CAD build for the part. Positions are in the model's coordinates, mm. Face numbers are marked on the shaded views. A direction names the side the tool comes from. Round coordinates to 2 decimals unless told otherwise and drop trailing zeros. Loops run counter-clockwise (first coordinate to the right, second up) from the corner with the lowest first, then second, coordinate; pieces in that order, holes last. Notation, with made-up numbers: M 76.5,-1.75 L 107.5,-1.75 A7 ccw 107.5,6.25 Z; hole C -27,32 d8. An arc over 180 degrees is marked long. Use a Markdown table: item, result. Add a question column.
(1) Wall check: L1, parallel to Y at x = -15.25, z = 1.2; L2, parallel to Y at x = 5.5, z = 7.75; L3, parallel to Z at x = 8, y = 13. Give the ranges that are in metal, low to high.
(2) Band-saw the part on D-D, the plane y = -9.5. Write the cut outline in (x, z), and give its area (3 significant figures).
(3) Which spindle directions (+Z, -Z, +X, -X, +Y, -Y) get a long thin tool onto all of the face, cutting with end or side? Do the marked faces 1, 2 and 3. Say none if no direction does.
(4) Band-saw the part on A-A, the plane x = 6.5. Give the number of separate pieces and of enclosed holes in the cut face, and give its area (3 significant figures).
(5) Flat gauge pins, fed straight in: P1, Ø1.5, axis at x = 8, z = 3.5, coming from the -Y side; P2, Ø1.6, axis at x = 15, z = 7.5, coming from the +Y side; P3, Ø2.5, axis at x = 15.25, y = -15.25, coming from the +Z side; P4, Ø3, axis at y = 10, z = 7.5, coming from the +X side. Where does each tip first touch, or does it go through?
(6) Band-saw the part on C-C, the plane y = -15.25. Write the cut outline in (x, z), and give its area (3 significant figures).
(7) Band-saw the part on B-B, the plane x = -15.25. Write the cut outline in (y, z), and give its area (3 significant figures).
(8) Two-plate mould, pull along Y, no slides. Class the marked faces 4, 5 and 6: released by +Y, released by -Y, zero draft, split by the parting line, or undercut.
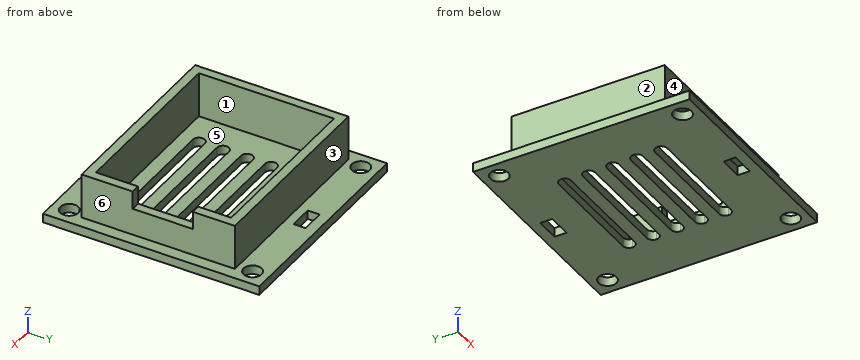
from build123d import *

# Parameters (mm, degrees)
F0_W      = 36
F0_H      = 36
F0_R      = 1.5
F3_DEPTH  = 1.5
F1_W      = 32
F1_H      = 25.5
F4_DEPTH  = 9
F5_T      = -1.5
F6_DEPTH  = 25
F7_W      = 1.5
F7_H      = 10
F8_DEPTH  = 3
F9_W      = 4
F9_H      = 2
F10_DEPTH = 25


with BuildPart() as f3:
    # F0 (on Top) → F3 (new body)
    with BuildSketch(Plane.XY):
        Rectangle(F0_W, F0_H)
        with Locations((-15.25, -15.25)):
            Circle(F0_R, mode=Mode.SUBTRACT)
        with Locations((15.25, -15.25)):
            Circle(F0_R, mode=Mode.SUBTRACT)
        with Locations((-15.25, 15.25)):
            Circle(F0_R, mode=Mode.SUBTRACT)
        with Locations((15.25, 15.25)):
            Circle(F0_R, mode=Mode.SUBTRACT)
    extrude(amount=F3_DEPTH)

    # F1 (on Top) → F4 (join)
    with BuildSketch(Plane.XY):
        Rectangle(F1_W, F1_H)
    extrude(amount=F4_DEPTH)

    # F5
    f5_openings = [f3.faces().sort_by_distance(p)[0] for p in [
        (0, 0, 9),
    ]]
    offset(amount=F5_T, openings=f5_openings, kind=Kind.INTERSECTION)

    # F2 (on Top) → F6 (cut)
    with BuildSketch(Plane.XY):
        with BuildLine():
            ThreePointArc((-8, 0), (-8.2928932188, 0.7071067812), (-9, 1))
            Line((-9, 1), (-9, -1))
            ThreePointArc((-9, -1), (-8.2928932188, -0.7071067812), (-8, 0))
        make_face()
        with BuildLine():
            Line((9, 1), (-9, 1))
            ThreePointArc((-9, 1), (-8.2928932188, 0.7071067812), (-8, 0))
            ThreePointArc((-8, 0), (-8.2928932188, -0.7071067812), (-9, -1))
            Line((-9, -1), (9, -1))
            ThreePointArc((9, -1), (8, 0), (9, 1))
        make_face()
        with BuildLine():
            Line((-9, -1), (-9, 1))
            ThreePointArc((-9, 1), (-10, 0), (-9, -1))
        make_face()
        with BuildLine():
            ThreePointArc((10, 0), (9.7071067812, 0.7071067812), (9, 1))
            Line((9, 1), (9, -1))
            ThreePointArc((9, -1), (9.7071067812, -0.7071067812), (10, 0))
        make_face()
        with BuildLine():
            Line((9, -1), (9, 1))
            ThreePointArc((9, 1), (8, 0), (9, -1))
        make_face()
        with BuildLine():
            ThreePointArc((-8, 4), (-8.2928932188, 3.2928932188), (-9, 3))
            Line((-9, 3), (9, 3))
            ThreePointArc((9, 3), (8, 4), (9, 5))
            Line((9, 5), (-9, 5))
            ThreePointArc((-9, 5), (-8.2928932188, 4.7071067812), (-8, 4))
        make_face()
        with BuildLine():
            Line((-9, 5), (-9, 3))
            ThreePointArc((-9, 3), (-8.2928932188, 3.2928932188), (-8, 4))
            ThreePointArc((-8, 4), (-8.2928932188, 4.7071067812), (-9, 5))
        make_face()
        with BuildLine():
            ThreePointArc((-9, 5), (-10, 4), (-9, 3))
            Line((-9, 3), (-9, 5))
        make_face()
        with BuildLine():
            Line((9, 5), (9, 3))
            ThreePointArc((9, 3), (9.7071067812, 3.2928932188), (10, 4))
            ThreePointArc((10, 4), (9.7071067812, 4.7071067812), (9, 5))
        make_face()
        with BuildLine():
            ThreePointArc((9, 5), (8, 4), (9, 3))
            Line((9, 3), (9, 5))
        make_face()
        with BuildLine():
            ThreePointArc((-8, 8), (-8.2928932188, 7.2928932188), (-9, 7))
            Line((-9, 7), (9, 7))
            ThreePointArc((9, 7), (8, 8), (9, 9))
            Line((9, 9), (-9, 9))
            ThreePointArc((-9, 9), (-8.2928932188, 8.7071067812), (-8, 8))
        make_face()
        with BuildLine():
            Line((-9, 9), (-9, 7))
            ThreePointArc((-9, 7), (-8.2928932188, 7.2928932188), (-8, 8))
            ThreePointArc((-8, 8), (-8.2928932188, 8.7071067812), (-9, 9))
        make_face()
        with BuildLine():
            ThreePointArc((-9, 9), (-10, 8), (-9, 7))
            Line((-9, 7), (-9, 9))
        make_face()
        with BuildLine():
            Line((9, 9), (9, 7))
            ThreePointArc((9, 7), (9.7071067812, 7.2928932188), (10, 8))
            ThreePointArc((10, 8), (9.7071067812, 8.7071067812), (9, 9))
        make_face()
        with BuildLine():
            ThreePointArc((9, 9), (8, 8), (9, 7))
            Line((9, 7), (9, 9))
        make_face()
        with BuildLine():
            ThreePointArc((9, -5), (9.7071067812, -4.7071067812), (10, -4))
            ThreePointArc((10, -4), (9.7071067812, -3.2928932188), (9, -3))
            Line((9, -3), (9, -5))
        make_face()
        with BuildLine():
            Line((9, -5), (9, -3))
            ThreePointArc((9, -3), (8, -4), (9, -5))
        make_face()
        with BuildLine():
            ThreePointArc((9, -5), (8, -4), (9, -3))
            Line((9, -3), (-9, -3))
            ThreePointArc((-9, -3), (-8.2928932188, -3.2928932188), (-8, -4))
            ThreePointArc((-8, -4), (-8.2928932188, -4.7071067812), (-9, -5))
            Line((-9, -5), (9, -5))
        make_face()
        with BuildLine():
            Line((-9, -5), (-9, -3))
            ThreePointArc((-9, -3), (-10, -4), (-9, -5))
        make_face()
        with BuildLine():
            ThreePointArc((-8, -4), (-8.2928932188, -3.2928932188), (-9, -3))
            Line((-9, -3), (-9, -5))
            ThreePointArc((-9, -5), (-8.2928932188, -4.7071067812), (-8, -4))
        make_face()
        with BuildLine():
            ThreePointArc((9, -9), (9.7071067812, -8.7071067812), (10, -8))
            ThreePointArc((10, -8), (9.7071067812, -7.2928932188), (9, -7))
            Line((9, -7), (9, -9))
        make_face()
        with BuildLine():
            Line((9, -9), (9, -7))
            ThreePointArc((9, -7), (8, -8), (9, -9))
        make_face()
        with BuildLine():
            ThreePointArc((9, -9), (8, -8), (9, -7))
            Line((9, -7), (-9, -7))
            ThreePointArc((-9, -7), (-8.2928932188, -7.2928932188), (-8, -8))
            ThreePointArc((-8, -8), (-8.2928932188, -8.7071067812), (-9, -9))
            Line((-9, -9), (9, -9))
        make_face()
        with BuildLine():
            Line((-9, -9), (-9, -7))
            ThreePointArc((-9, -7), (-10, -8), (-9, -9))
        make_face()
        with BuildLine():
            ThreePointArc((-8, -8), (-8.2928932188, -7.2928932188), (-9, -7))
            Line((-9, -7), (-9, -9))
            ThreePointArc((-9, -9), (-8.2928932188, -8.7071067812), (-8, -8))
        make_face()
    extrude(amount=F6_DEPTH, mode=Mode.SUBTRACT)

    # F7 (on face) → F8 (cut)
    with BuildSketch(Plane.XY.offset(9)):
        with Locations((15.25, 0.75)):
            Rectangle(F7_W, F7_H)
    extrude(amount=-F8_DEPTH, mode=Mode.SUBTRACT)

    # F9 (on face) → F10 (cut)
    with BuildSketch(Plane.XY.offset(1.5)):
        with Locations((0, 15.25)):
            Rectangle(F9_W, F9_H)
        with Locations((0, -15.25)):
            Rectangle(F9_W, F9_H)
    extrude(amount=-F10_DEPTH, mode=Mode.SUBTRACT)


solid = f3.part
Return value:
| question | item | result |
|---|---|---|
| 1 | L1 | -18 to -16.75, -13.75 to 13.75, 16.75 to 18 |
| 1 | L2 | -12.75 to -11.25, 11.25 to 12.75 |
| 1 | L3 | 0 to 1.5 |
| 2 | outline | M -18,0 L 18,0 L 18,1.5 L 16,1.5 L 16,9 L 14.5,9 L 14.5,1.5 L -14.5,1.5 L -14.5,9 L -16,9 L -16,1.5 L -18,1.5 Z |
| 2 | area | 76.5 mm^2 |
| 3 | face 1 | +Z |
| 3 | face 2 | +Z, -X, +Y, -Y |
| 3 | face 3 | +Z, +X, -X, +Y |
| 4 | separate pieces | 6 |
| 4 | enclosed holes | 0 |
| 4 | area | 61.5 mm^2 |
| 5 | P1 | y = -12.75 |
| 5 | P2 | y = 12.75 |
| 5 | P3 | through |
| 5 | P4 | x = 16 |
| 6 | outline | M -18,0 L -16.75,0 L -16.75,1.5 L -18,1.5 Z; M -13.75,0 L -2,0 L -2,1.5 L -13.75,1.5 Z; M 2,0 L 13.75,0 L 13.75,1.5 L 2,1.5 Z; M 16.75,0 L 18,0 L 18,1.5 L 16.75,1.5 Z |
| 6 | area | 39.0 mm^2 |
| 7 | outline | M -18,0 L -16.75,0 L -16.75,1.5 L -18,1.5 Z; M -13.75,0 L 13.75,0 L 13.75,1.5 L 12.75,1.5 L 12.75,9 L -12.75,9 L -12.75,1.5 L -13.75,1.5 Z; M 16.75,0 L 18,0 L 18,1.5 L 16.75,1.5 Z |
| 7 | area | 236 mm^2 |
| 8 | face 4 | released by -Y |
| 8 | face 5 | undercut |
| 8 | face 6 | zero draft |
